Read the model definition and answer for the solid it produces. Units are mm, in the model's axes. A direction names the side the tool comes from. Give positions to 0.01 mm unless a question says otherwise; leave off trailing zeros. Put each result on its own line as item: value. Start each with the question number.
from build123d import *

# Parameters (mm, degrees)
SKETCH1_R           = 2.1
BOSS_EXTRUDE1_DEPTH = 275
FILLET1_R           = 1


with BuildPart() as part:
    # Sketch1 → Boss-Extrude1 (new body)
    with BuildSketch(Plane.XY):
        with BuildLine():
            Line((-2.839339828, 3.9), (-5.470710678, 6.53137085))
            ThreePointArc((-5.470710678, 6.53137085), (-5.492387953, 6.563813185), (-5.5, 6.602081528))
            Line((-5.5, 6.602081528), (-5.5, 8.1))
            ThreePointArc((-5.5, 8.1), (-5.470710678, 8.170710678), (-5.4, 8.2))
            Line((-5.4, 8.2), (-3.334418044, 8.2))
            ThreePointArc((-3.334418044, 8.2), (-3.244178397, 8.256909326), (-3.2566483, 8.362863876))
            Line((-3.2566483, 8.362863876), (-4.58, 10))
            Line((-4.58, 10), (-10, 10))
            Line((-10, 10), (-10, 4.58))
            Line((-10, 4.58), (-8.362863876, 3.2566483))
            ThreePointArc((-8.362863876, 3.2566483), (-8.256909326, 3.244178397), (-8.2, 3.334418044))
            Line((-8.2, 3.334418044), (-8.2, 5.4))
            ThreePointArc((-8.2, 5.4), (-8.170710678, 5.470710678), (-8.1, 5.5))
            Line((-8.1, 5.5), (-6.602081528, 5.5))
            ThreePointArc((-6.602081528, 5.5), (-6.563813185, 5.492387953), (-6.53137085, 5.470710678))
            Line((-6.53137085, 5.470710678), (-3.9, 2.839339828))
            Line((-3.9, 2.839339828), (-3.9, -2.839339828))
            Line((-3.9, -2.839339828), (-6.53137085, -5.470710678))
            ThreePointArc((-6.53137085, -5.470710678), (-6.563813185, -5.492387953), (-6.602081528, -5.5))
            Line((-6.602081528, -5.5), (-8.1, -5.5))
            ThreePointArc((-8.1, -5.5), (-8.170710678, -5.470710678), (-8.2, -5.4))
            Line((-8.2, -5.4), (-8.2, -3.334418044))
            ThreePointArc((-8.2, -3.334418044), (-8.256909326, -3.244178397), (-8.362863876, -3.2566483))
            Line((-8.362863876, -3.2566483), (-10, -4.58))
            Line((-10, -4.58), (-10, -10))
            Line((-10, -10), (-4.58, -10))
            Line((-4.58, -10), (-3.2566483, -8.362863876))
            ThreePointArc((-3.2566483, -8.362863876), (-3.244178397, -8.256909326), (-3.334418044, -8.2))
            Line((-3.334418044, -8.2), (-5.4, -8.2))
            ThreePointArc((-5.4, -8.2), (-5.470710678, -8.170710678), (-5.5, -8.1))
            Line((-5.5, -8.1), (-5.5, -6.602081528))
            ThreePointArc((-5.5, -6.602081528), (-5.492387953, -6.563813185), (-5.470710678, -6.53137085))
            Line((-5.470710678, -6.53137085), (-2.839339828, -3.9))
            Line((-2.839339828, -3.9), (2.839339828, -3.9))
            Line((2.839339828, -3.9), (5.470710678, -6.53137085))
            ThreePointArc((5.470710678, -6.53137085), (5.492387953, -6.563813185), (5.5, -6.602081528))
            Line((5.5, -6.602081528), (5.5, -8.1))
            ThreePointArc((5.5, -8.1), (5.470710678, -8.170710678), (5.4, -8.2))
            Line((5.4, -8.2), (3.334418044, -8.2))
            ThreePointArc((3.334418044, -8.2), (3.244178397, -8.256909326), (3.2566483, -8.362863876))
            Line((3.2566483, -8.362863876), (4.58, -10))
            Line((4.58, -10), (10, -10))
            Line((10, -10), (10, -4.58))
            Line((10, -4.58), (8.362863876, -3.2566483))
            ThreePointArc((8.362863876, -3.2566483), (8.256909326, -3.244178397), (8.2, -3.334418044))
            Line((8.2, -3.334418044), (8.2, -5.4))
            ThreePointArc((8.2, -5.4), (8.170710678, -5.470710678), (8.1, -5.5))
            Line((8.1, -5.5), (6.602081528, -5.5))
            ThreePointArc((6.602081528, -5.5), (6.563813185, -5.492387953), (6.53137085, -5.470710678))
            Line((6.53137085, -5.470710678), (3.9, -2.839339828))
            Line((3.9, -2.839339828), (3.9, 2.839339828))
            Line((3.9, 2.839339828), (6.53137085, 5.470710678))
            ThreePointArc((6.53137085, 5.470710678), (6.563813185, 5.492387953), (6.602081528, 5.5))
            Line((6.602081528, 5.5), (8.1, 5.5))
            ThreePointArc((8.1, 5.5), (8.170710678, 5.470710678), (8.2, 5.4))
            Line((8.2, 5.4), (8.2, 3.334418044))
            ThreePointArc((8.2, 3.334418044), (8.256909326, 3.244178397), (8.362863876, 3.2566483))
            Line((8.362863876, 3.2566483), (10, 4.58))
            Line((10, 4.58), (10, 10))
            Line((10, 10), (4.58, 10))
            Line((4.58, 10), (3.2566483, 8.362863876))
            ThreePointArc((3.2566483, 8.362863876), (3.244178397, 8.256909326), (3.334418044, 8.2))
            Line((3.334418044, 8.2), (5.4, 8.2))
            ThreePointArc((5.4, 8.2), (5.470710678, 8.170710678), (5.5, 8.1))
            Line((5.5, 8.1), (5.5, 6.602081528))
            ThreePointArc((5.5, 6.602081528), (5.492387953, 6.563813185), (5.470710678, 6.53137085))
            Line((5.470710678, 6.53137085), (2.839339828, 3.9))
            Line((2.839339828, 3.9), (-2.839339828, 3.9))
        make_face()
        Circle(SKETCH1_R, mode=Mode.SUBTRACT)
    extrude(amount=BOSS_EXTRUDE1_DEPTH)

    # Fillet1
    fillet1_edges = [part.edges().sort_by_distance(p)[0] for p in [
        (10, -10, 137.5),
        (-10, -10, 137.5),
        (-10, 10, 137.5),
        (10, 10, 137.5),
    ]]
    fillet(fillet1_edges, radius=FILLET1_R)


solid = part.part
1) Each of these flat-tipped pins is pushed along its axis until it touches: pin 1 Ø1 at (x, z) = (-2, 224.5) entering from +Y; pin 2 Ø4.5 at (y, z) = (0, 199) entering from +X; pin 3 Ø1 at (y, z) = (-4, 83) entering from -X. Where does it stop, or does it pass through?
2) For a pull along Y with two mould halves and no side action, classify faces 4 (the face through (7, -10, 136)), 5 (the face through (0, 3.9, 136)), 6 (the face through (3.9, 0, 136)) as pulls with the +Y half, pulls with the -Y half, needs draft (parallel to the pull), parting line crosses it, or undercut.
3) For faces 1 (the face through (-3.9, 0, 136)), 2 (the face through (-7, 10, 136)), 3 (the face through (0, -3.9, 136)), determine the directions among +Z, -Z, +X, -X, +Y, -Y from which every point of the face is accessible in a straight line to the end or side of a thin tool.
4) Straight lines are drawn through the part: line 1 (X direction, y = 8.25, z = 132.5); line 2 (Y direction, x = -4.25, z = 98); line 3 (Y direction, x = 0, z = 106). For each, find the intervals that lie inside material, in ascending order. Write a range as [from, to].
Results found:
1. pin 1: stops at y = 3.9
1. pin 2: stops at x = 3.9
1. pin 3: stops at x = -9.9
2. face 4: pulls with the -Y half
2. face 5: pulls with the +Y half
2. face 6: undercut
3. face 1: +Z, -Z, -X
3. face 2: +Z, -Z, +X, -X, +Y
3. face 3: +Z, -Z, -Y
4. line 1: x = [-10, -3.25], [3.25, 10]
4. line 2: y = [-9.59, -8.2], [-5.31, -3.19], [3.19, 5.31], [8.2, 9.59]
4. line 3: y = [-3.9, -2.1], [2.1, 3.9]
